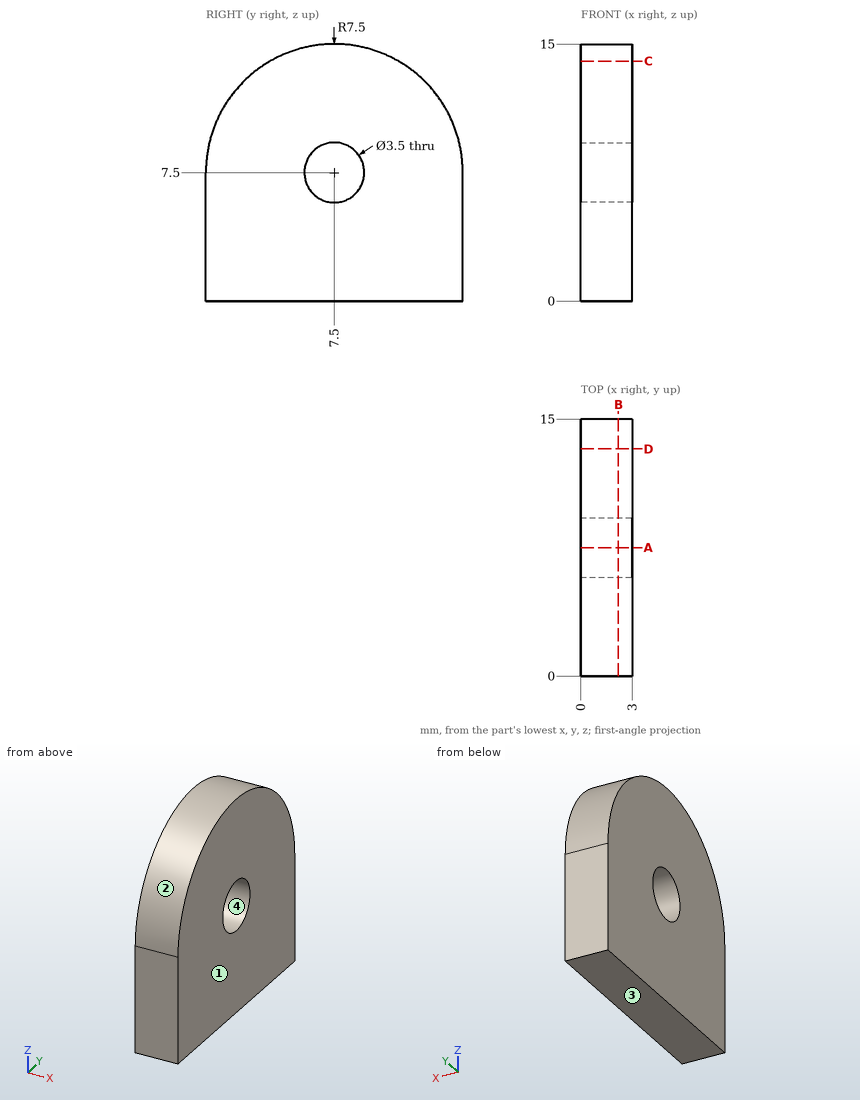
Design review of the part shown in the three views and the two pictorial views. Dimensions are in mm from the part's minimum x, y and z. Give positions to 0.01 mm unless a question says otherwise; leave off trailing zeros. Write each loop counter-clockwise with the first axis right and the second up, starting at its lowest first coordinate (ties: lowest second). Pieces come first, ordered by that corner, then holes.
(1) Add section A-A (y = 7.5). Give the boundary of the cut face in (x, z).
Checked values:
outline: (0, 0) - (3, 0) - (3, 5.75) - (0, 5.75) - close; (0, 9.25) - (3, 9.25) - (3, 15) - (0, 15) - close
(2) Wall thickness on line 1 along Y through (x, z) = (0.9, 7.5); line 2 along Z through (x, y) = (1.7, 8); line 3 along Z through (x, y) = (1.55, 6): over which ranges is each line inside the solid? List them lowest first.
Checked values:
line 1: y = 0 to 5.75, 9.25 to 15
line 2: z = 0 to 5.82, 9.18 to 14.98
line 3: z = 0 to 6.6, 8.4 to 14.85
(3) Add section B-B (x = 2.2). Give the boundary of the cut face in (y, z).
Checked values:
outline: (0, 0) - (15, 0) - (15, 7.5) arc R7.5 ccw to (0, 7.5) - close; hole circle Ø3.5 at (7.5, 7.5)
(4) Add section D-D (y = 13.25). Give the boundary of the cut face in (x, z).
Checked values:
outline: (0, 0) - (3, 0) - (3, 12.32) - (0, 12.32) - close
(5) Mouldability with a two-part tool opening along Z and no side actions: class the marked faces 1, 2, 3 and 4 as +Z half, -Z half, draft (parallel to the pull), parting line (faces both ways), or undercut.
Checked values:
face 1: draft
face 2: +Z half
face 3: -Z half
face 4: undercut
(6) Add section C-C (z = 14). Give the boundary of the cut face in (x, y).
Checked values:
outline: (0, 3.76) - (3, 3.76) - (3, 11.24) - (0, 11.24) - close
(7) Clearance check with flat-ended pins moving along their axes: pin 1 Ø1 at (x, z) = (2, 13.5) entering from +Y; pin 2 Ø2 at (y, z) = (4.5, 2.5) entering from -X. State where each tip first meets the part, or that it passes through.
Checked values:
pin 1: stops at y = 12.6
pin 2: stops at x = 0
